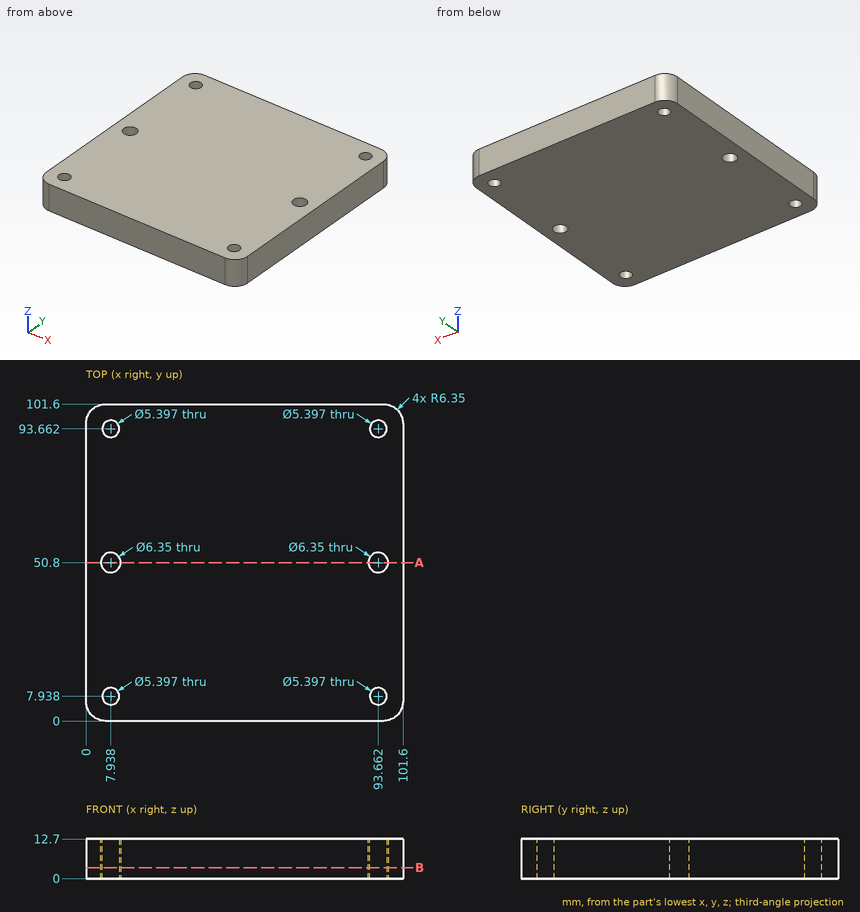
The figure shows three views and two pictorial views of one solid part (mm, origin at its lowest corner). Answer the questions. Give positions to 0.01 mm unless a question says otherwise; leave off trailing zeros. Loops run counter-clockwise (first coordinate to the right, second up) from the corner with the lowest first, then second, coordinate; pieces in that order, holes last. Notation, with made-up numbers: (38.5, 49) - (97.5, 49) arc R24 cw to (97.5, 61) - close; hole circle Ø3 at (-16.75, -30). An arc over 180 degrees is marked (long way). Use one line per item in the form item = value.
1. Section A-A on y = 50.8 is taken. Give the vertices of the cut face in (x, z).
Calculated:
outline = (0, 0) - (4.76, 0) - (4.76, 12.7) - (0, 12.7) - close; (11.11, 0) - (90.49, 0) - (90.49, 12.7) - (11.11, 12.7) - close; (96.84, 0) - (101.6, 0) - (101.6, 12.7) - (96.84, 12.7) - close
2. Given pin 1 Ø5 at (x, y) = (93.66, 93.66) entering from -Z, flat-ended and moving along its own axis, determine where the tip first touches the part or whether it passes through.
Calculated:
pin_1 = through
3. Section B-B on z = 3.5 is taken. Count the separate pieces of the cut face and the enclosed holes in it, then the cut area to 3 significant figures.
Calculated:
separate_pieces = 1
enclosed_holes = 6
area = 10,100 mm^2
4. Find the intervals of material crossed by line 1 along X through (y, z) = (52.5, 10.25) (1 decimal); line 2 along Y through (x, z) = (92.5, 11) (1 decimal), in increasing order. Write a range as [from, to].
Calculated:
line_1 = [0, 5.3], [10.6, 91], [96.3, 101.6]
line_2 = [0, 5.5], [10.4, 47.8], [53.8, 91.2], [96.1, 101.6]
